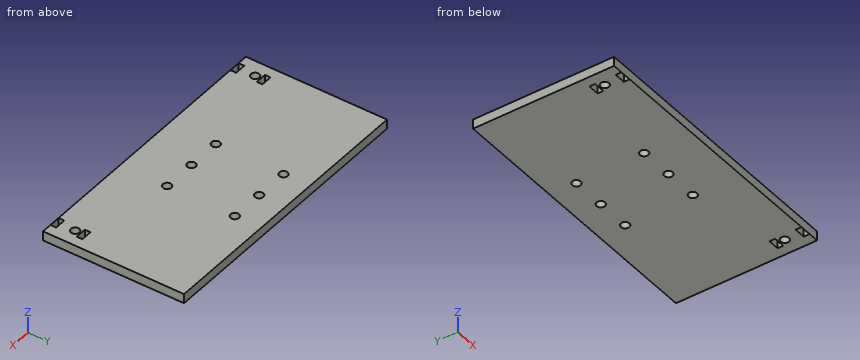
```python
from build123d import *

# Parameters (mm, degrees)
ESQUISSE1_W        = 150
ESQUISSE1_H        = 75
ESQUISSE1_R        = 2.25
ESQUISSE1_W_2      = 6
ESQUISSE1_H_2      = 3
BOSS_EXTRU_1_DEPTH = 5


with BuildPart() as part:
    # Esquisse1 → Boss.-Extru.1 (new body)
    with BuildSketch(Plane.XY):
        with Locations((75, -37.5)):
            Rectangle(ESQUISSE1_W, ESQUISSE1_H)
        with Locations((8.5, -64)):
            Circle(ESQUISSE1_R, mode=Mode.SUBTRACT)
        with Locations((141.5, -64)):
            Circle(ESQUISSE1_R, mode=Mode.SUBTRACT)
        with Locations((57, -14)):
            Circle(ESQUISSE1_R, mode=Mode.SUBTRACT)
        with Locations((93, -14)):
            Circle(ESQUISSE1_R, mode=Mode.SUBTRACT)
        with Locations((93, -50)):
            Circle(ESQUISSE1_R, mode=Mode.SUBTRACT)
        with Locations((57, -50)):
            Circle(ESQUISSE1_R, mode=Mode.SUBTRACT)
        with Locations((75, -14)):
            Circle(ESQUISSE1_R, mode=Mode.SUBTRACT)
        with Locations((75, -50)):
            Circle(ESQUISSE1_R, mode=Mode.SUBTRACT)
        with Locations((8.5, -59.5)):
            Rectangle(ESQUISSE1_W_2, ESQUISSE1_H_2, mode=Mode.SUBTRACT)
        with Locations((8.5, -73.4)):
            Rectangle(ESQUISSE1_W_2, ESQUISSE1_H_2, mode=Mode.SUBTRACT)
        with Locations((141.5, -59.5)):
            Rectangle(ESQUISSE1_W_2, ESQUISSE1_H_2, mode=Mode.SUBTRACT)
        with Locations((141.5, -73.4)):
            Rectangle(ESQUISSE1_W_2, ESQUISSE1_H_2, mode=Mode.SUBTRACT)
    extrude(amount=BOSS_EXTRU_1_DEPTH)


solid = part.part
```
Model file for the job. Use its own axes, mm. Round coordinates to 2 decimals unless told otherwise and drop trailing zeros. Write each loop counter-clockwise with the first axis right and the second up, starting at its lowest first coordinate (ties: lowest second). Pieces come first, ordered by that corner, then holes. Notation, with made-up numbers: (17.25, -7.5) - (49.25, -7.5) arc R17 ccw to (49.25, 22.5) - close; hole circle Ø5 at (57, 14). An arc over 180 degrees is marked (long way). One line per item, written item: value.
(1) Cut at A-A, the plane y = -50. Give the cut face in (x, z), plus the area to 4 significant figures.
Values follow:
outline: (0, 0) - (54.75, 0) - (54.75, 5) - (0, 5) - close; (59.25, 0) - (72.75, 0) - (72.75, 5) - (59.25, 5) - close; (77.25, 0) - (90.75, 0) - (90.75, 5) - (77.25, 5) - close; (95.25, 0) - (150, 0) - (150, 5) - (95.25, 5) - close
area: 682.5 mm²
(2) Wall check: probe 1 along Y at (x, z) = (75, 2.2); probe 2 along X at (y, z) = (-13, 2.45); probe 3 along Y at (x, z) = (92, 0.5). Give the ranges that are in metal, low to high.
Values follow:
probe 1: y = -75 to -52.25, -47.75 to -16.25, -11.75 to 0
probe 2: x = 0 to 54.98, 59.02 to 72.98, 77.02 to 90.98, 95.02 to 150
probe 3: y = -75 to -52.02, -47.98 to -16.02, -11.98 to 0
(3) Cut at B-B, the plane x = 141.5. Give the cut face in (y, z).
Values follow:
outline: (-75, 0) - (-74.9, 0) - (-74.9, 5) - (-75, 5) - close; (-71.9, 0) - (-66.25, 0) - (-66.25, 5) - (-71.9, 5) - close; (-61.75, 0) - (-61, 0) - (-61, 5) - (-61.75, 5) - close; (-58, 0) - (0, 0) - (0, 5) - (-58, 5) - close
(4) Cut at C-C, the plane z = 1. Give the number of separate pieces and of enclosed holes in the cut face, plus the area to 3 significant figures.
Values follow:
separate pieces: 1
enclosed holes: 12
area: 11,100 mm²
(5) Cut at D-D, the plane x = 75. Give the cut face in (y, z).
Values follow:
outline: (-75, 0) - (-52.25, 0) - (-52.25, 5) - (-75, 5) - close; (-47.75, 0) - (-16.25, 0) - (-16.25, 5) - (-47.75, 5) - close; (-11.75, 0) - (0, 0) - (0, 5) - (-11.75, 5) - close
